CAD build for the part. Positions are in the model's coordinates, mm. A direction names the side the tool comes from. Round coordinates to 2 decimals unless told otherwise and drop trailing zeros. Loops run counter-clockwise (first coordinate to the right, second up) from the corner with the lowest first, then second, coordinate; pieces in that order, holes last. Notation, with made-up numbers: M 55.5,60.5 L 113.5,60.5 A24 ccw 113.5,99.5 Z; hole C 52.25,40.25 d6. An arc over 180 degrees is marked long. Use a Markdown table: item, result. Add a question column.
(1) Band-saw the part on A-A, the plane x = 0. Write the cut outline in (y, z).
(2) Two-plate mould, pull along Y, no slides. Class faces 1 (the face through (0, 8, 8)), 2 (the face through (95.38, 30.04, 2.46)), 3 (the face through (0, -8, 8)), 4 (the face through (-1, -19, 15)): released by +Y, released by -Y, zero draft, split by the parting line, or undercut.
(3) Band-saw the part on B-B, the plane y = 0. Write the cut outline in (x, z), and give its area (3 significant figures).
(4) Wall check: L1, parallel to Y at x = 0.5, z = 1.25; L2, parallel to Y at x = 0, z = 13.5; L3, parallel to X at y = 57, z = 13.5. Give the ranges that are in metal, low to high.
(5) Which spindle directions (+Z, -Z, +X, -X, +Y, -Y) get a long thin tool onto all of the face, cutting with end or side? Do faces 5 (the face through (10, 0, 8)), 6 (the face through (-1, -21, 0)). Say none if no direction does.
(6) Flat gauge pins, fed straight in: P1, Ø6, axis at y = 47, z = 4.5, coming from the -X side; P2, Ø1.5, axis at x = 47.5, z = 11, coming from the -Y side; P3, Ø2, axis at x = -19.5, z = 2.5, coming from the -Y side. Where does each tip first touch, or does it go through?
(7) Band-saw the part on C-C, the plane z = 8.75. Write the cut outline in (x, y), and give its area (3 significant figures).
from build123d import *

# Parameters (mm, degrees)
F0_R     = 100
F1_DEPTH = 15
F2_R     = 10
F3_W     = 20
F3_H     = 16
F4_DEPTH = 50


with BuildPart() as f1:
    # F0 (on Top) → F1 (new body)
    with BuildSketch(Plane.XY):
        Circle(F0_R)
    extrude(amount=F1_DEPTH)

    # F2
    f2_edges = [f1.edges().sort_by_distance(p)[0] for p in [
        (-100, 0, 15),
    ]]
    fillet(f2_edges, radius=F2_R)

    # F3 (on face) → F4 (cut)
    with BuildSketch(Plane.XY.offset(15)):
        Rectangle(F3_W, F3_H)
    extrude(amount=-F4_DEPTH, mode=Mode.SUBTRACT)


solid = f1.part
Return value:
| question | item | result |
|---|---|---|
| 1 | outline | M -100,0 L -8,0 L -8,15 L -90,15 A10 ccw -100,5 Z; M 8,0 L 100,0 L 100,5 A10 ccw 90,15 L 8,15 Z |
| 2 | face 1 | undercut |
| 2 | face 2 | split by the parting line |
| 2 | face 3 | undercut |
| 2 | face 4 | zero draft |
| 3 | outline | M -100,0 L -10,0 L -10,15 L -90,15 A10 ccw -100,5 Z; M 10,0 L 100,0 L 100,5 A10 ccw 90,15 L 10,15 Z |
| 3 | area | 2,660 mm^2 |
| 4 | L1 | -100 to -8, 8 to 100 |
| 4 | L2 | -95.27 to -8, 8 to 95.27 |
| 4 | L3 | -76.33 to 76.33 |
| 5 | face 5 | +Z, -Z |
| 5 | face 6 | -Z, +X, -X, +Y, -Y |
| 6 | P1 | x = -89.8 |
| 6 | P2 | y = -86.44 |
| 6 | P3 | y = -98.27 |
| 7 | outline | C 0,0 d198.54; hole M -10,-8 L 10,-8 L 10,8 L -10,8 Z |
| 7 | area | 30,600 mm^2 |
